Read the model definition and answer for the solid it produces. Units are mm, in the model's axes. A direction names the side the tool comes from. Coordinates: 2 decimals unless noted, no trailing zeros. Loops run counter-clockwise (first coordinate to the right, second up) from the corner with the lowest first, then second, coordinate; pieces in that order, holes last. Notation, with made-up numbers: M -32.5,44 L 16.5,44 A28 cw 16.5,74 Z; hole C -27,13.25 d5. An arc over 180 degrees is marked long. Put each result on its own line as item: value.
from build123d import *

# Parameters (mm, degrees)
ESQUISSE1_R             = 48.5
BOSS_EXTRU_1_DEPTH      = 44
ESQUISSE2_R             = 48.5
ESQUISSE2_R_2           = 47
ENL_V_MAT_EXTRU_1_DEPTH = 6
ESQUISSE3_R             = 35
ENL_V_MAT_EXTRU_2_DEPTH = 45
ESQUISSE5_R             = 45.5
ESQUISSE5_R_2           = 36.5
ENL_V_MAT_EXTRU_3_DEPTH = 42
ESQUISSE6_W             = 20
ESQUISSE6_H             = 4.166829754
ENL_V_MAT_EXTRU_5_DEPTH = 42
BOSS_EXTRU_2_DEPTH      = 6


with BuildPart() as part:
    # Esquisse1 → Boss.-Extru.1 (new body)
    with BuildSketch(Plane.XY):
        Circle(ESQUISSE1_R)
    extrude(amount=BOSS_EXTRU_1_DEPTH)

    # Esquisse2 → Enlèv. mat.-Extru.1 (cut)
    with BuildSketch(Plane.XY.offset(44)):
        Circle(ESQUISSE2_R)
        Circle(ESQUISSE2_R_2, mode=Mode.SUBTRACT)
    extrude(amount=-ENL_V_MAT_EXTRU_1_DEPTH, mode=Mode.SUBTRACT)

    # Esquisse3 → Enlèv. mat.-Extru.2 (cut, through all)
    with BuildSketch(Plane.XY.offset(44)):
        Circle(ESQUISSE3_R)
    extrude(amount=-ENL_V_MAT_EXTRU_2_DEPTH, mode=Mode.SUBTRACT)

    # Esquisse5 → Enlèv. mat.-Extru.3 (cut)
    with BuildSketch(Plane(origin=(0, 0, 0), x_dir=(-1, 0, 0), z_dir=(0, 0, -1))):
        Circle(ESQUISSE5_R)
        Circle(ESQUISSE5_R_2, mode=Mode.SUBTRACT)
    extrude(amount=-ENL_V_MAT_EXTRU_3_DEPTH, mode=Mode.SUBTRACT)

    # Esquisse6 → Enlèv. mat.-Extru.5 (cut)
    with BuildSketch(Plane(origin=(0, 0, 0), x_dir=(-1, 0, 0), z_dir=(0, 0, -1))):
        with Locations((0, -46.470913117)):
            Rectangle(ESQUISSE6_W, ESQUISSE6_H)
    extrude(amount=-ENL_V_MAT_EXTRU_5_DEPTH, mode=Mode.SUBTRACT)

    # Esquisse8 → Boss.-Extru.2 (add)
    with BuildSketch(Plane(origin=(0, 0, 0), x_dir=(-1, 0, 0), z_dir=(0, 0, -1))):
        with BuildLine():
            ThreePointArc((34.294678888, -34.294678888), (48.5, 0), (34.294678888, 34.294678888))
            Line((34.294678888, 34.294678888), (32.173358544, 32.173358544))
            ThreePointArc((32.173358544, 32.173358544), (45.5, 0), (32.173358544, -32.173358544))
            Line((32.173358544, -32.173358544), (34.294678888, -34.294678888))
        make_face()
        with BuildLine():
            ThreePointArc((-34.294678888, -34.294678888), (-48.5, 0), (-34.294678888, 34.294678888))
            Line((-34.294678888, 34.294678888), (-32.173358544, 32.173358544))
            ThreePointArc((-32.173358544, 32.173358544), (-45.5, 0), (-32.173358544, -32.173358544))
            Line((-32.173358544, -32.173358544), (-34.294678888, -34.294678888))
        make_face()
    extrude(amount=BOSS_EXTRU_2_DEPTH)


solid = part.part
1) Determine the mould class of faces 5 (the flat face through (19, -30, 0)), 6 (the cylindrical face through (44.83, 14.12, 41.04)), 7 (the flat face through (10, -46, 21)), 8 (the flat face through (46, 0, -6)) for opening direction X: released by +X, released by -X, zero draft, split by the parting line, or undercut.
Answer list:
face 5: undercut
face 6: split by the parting line
face 7: undercut
face 8: zero draft
2) Given pin 1 Ø2.5 at (y, z) = (-45.5, 11.5) entering from -X; pin 2 Ø12 at (x, y) = (25.5, -39) entering from -Z; pin 3 Ø12 at (y, z) = (-8, 32) entering from +X, each flat-ended and moving along its own axis, determine where each tip first touches the part or whether it passes through.
Answer list:
pin 1: stops at x = -19.85
pin 2: stops at z = 0
pin 3: stops at x = 48.46
3) Find section A-A, the plane x = 0. Write down the section's boundary in (y, z).
Answer list:
outline: M -47,42 L -36.5,42 L -36.5,0 L -35,0 L -35,44 L -47,44 Z; M 35,0 L 36.5,0 L 36.5,42 L 45.5,42 L 45.5,0 L 48.5,0 L 48.5,38 L 47,38 L 47,44 L 35,44 Z
4) Find section C-C, the plane y = 0. Write down the section's boundary in (x, z).
Answer list:
outline: M -48.5,-6 L -45.5,-6 L -45.5,42 L -36.5,42 L -36.5,0 L -35,0 L -35,44 L -47,44 L -47,38 L -48.5,38 Z; M 35,0 L 36.5,0 L 36.5,42 L 45.5,42 L 45.5,-6 L 48.5,-6 L 48.5,38 L 47,38 L 47,44 L 35,44 Z
5) Find section B-B, the plane z = 27. Write down the section's boundary in (x, y), plus the area to 3 significant figures.
Answer list:
outline: C 0,0 d73; M -10,-47.46 L -10,-44.39 A45.5 cw long 10,-44.39 L 10,-47.46 A48.5 ccw long Z; hole C 0,0 d70
area: 1,160 mm^2
6) Straight lines are drawn through the part: line 1 (Y direction, x = 0, z = 4); line 2 (X direction, y = -10.5, z = 23.5); line 3 (X direction, y = 20.5, z = 26). For each, find the intervals that lie inside material, in ascending order. Write a range as [from, to].
Answer list:
line 1: y = [-36.5, -35], [35, 36.5], [45.5, 48.5]
line 2: x = [-47.35, -44.27], [-34.96, -33.39], [33.39, 34.96], [44.27, 47.35]
line 3: x = [-43.95, -40.62], [-30.2, -28.37], [28.37, 30.2], [40.62, 43.95]
7) Which of the six approach directions +Z, -Z, +X, -X, +Y, -Y give full straight-line access (tool end or side, diameter ignored) to faces 1 (the flat face through (-40, 26, 38)), 2 (the flat face through (-46, 0, -6)), 3 (the cylindrical face through (7.912, -35.632, 20.706)), 4 (the flat face through (-10, -46, 21))?
Answer list:
face 1: +Z
face 2: -Z, +X, -X, +Y, -Y
face 3: -Z
face 4: -Z, -Y
8) Find section D-D, the plane y = -42. Write down the section's boundary in (x, z), plus the area to 3 significant figures.
Answer list:
outline: M -24.25,0 L -17.5,0 L -17.5,42 L 17.5,42 L 17.5,0 L 24.25,0 L 24.25,38 L 21.1,38 L 21.1,44 L -21.1,44 L -21.1,38 L -24.25,38 Z
area: 626 mm^2
